CAD build for the part. Positions are in the model's coordinates, mm. Round coordinates to 2 decimals unless told otherwise and drop trailing zeros. Order: outer loops, then holes, each group sorted by start corner. A loop starts at its lowest first (then second) coordinate and runs counter-clockwise, first axis right, second up.
```python
from build123d import *

# Parameters (mm, degrees)
SKETCH2_W           = 73
SKETCH2_H           = 13
SKETCH2_R           = 3.9
SKETCH2_R_2         = 3.95
SKETCH2_R_3         = 4
SKETCH2_R_4         = 4.05
SKETCH2_R_5         = 4.1
SKETCH2_R_6         = 4.15
SKETCH2_R_7         = 4.2
BOSS_EXTRUDE1_DEPTH = 5
FILLET1_R           = 5


with BuildPart() as part:
    # Sketch2 → Boss-Extrude1 (new body)
    with BuildSketch(Plane(origin=(0, 0, 0), x_dir=(1, 0, 0), z_dir=(0, 1, 0))):
        with Locations((30, 0)):
            Rectangle(SKETCH2_W, SKETCH2_H)
        Circle(SKETCH2_R, mode=Mode.SUBTRACT)
        with Locations((10, 0)):
            Circle(SKETCH2_R_2, mode=Mode.SUBTRACT)
        with Locations((20, 0)):
            Circle(SKETCH2_R_3, mode=Mode.SUBTRACT)
        with Locations((30, 0)):
            Circle(SKETCH2_R_4, mode=Mode.SUBTRACT)
        with Locations((40, 0)):
            Circle(SKETCH2_R_5, mode=Mode.SUBTRACT)
        with Locations((50, 0)):
            Circle(SKETCH2_R_6, mode=Mode.SUBTRACT)
        with Locations((60, 0)):
            Circle(SKETCH2_R_7, mode=Mode.SUBTRACT)
    extrude(amount=BOSS_EXTRUDE1_DEPTH)

    # Fillet1
    fillet1_edges = [part.edges().sort_by_distance(p)[0] for p in [
        (-6.5, 2.5, -6.5),
        (-6.5, 2.5, 6.5),
    ]]
    fillet(fillet1_edges, radius=FILLET1_R)


solid = part.part
```
1. Cut at D-D, the plane x = 50. Write the cut outline in (y, z).
2. Cut at C-C, the plane y = 4. Write the cut outline in (x, z).
3. Cut at A-A, the plane x = 40. Write the cut outline in (y, z).
4. Cut at B-B, the plane z = -0.75. Give the number of separate pieces and of enclosed holes in the cut face, and give its area (3 significant figures).
5. Pin check, flat tips, straight feed: P1, Ø5, axis at x = 50, z = 0, coming from the -Y side (3 decimals); P2, Ø6, axis at x = 29.5, z = 3.5, coming from the +Y side. Stop position of each tip, or through.
6. Drill centre lines: line 1 (Z direction, x = 0, y = 3.3); line 2 (Z direction, x = 20, y = 1.55); line 3 (X direction, y = 4.6, z = -4.25). Where is each one in solid material? Low to high.
7. Mould opens along Z. For faces 1 (the face through (-5.07, 2.54, -5)), 2 (the face through (35.904, 2.465, -0.18)), 3 (the face through (29.5, 5, -4.4)) say: released by +Z, released by -Z, zero draft, split by the parting line, or undercut.
Outcome:
1. outline: (0, -6.5) - (5, -6.5) - (5, -4.15) - (0, -4.15) - close; (0, 4.15) - (5, 4.15) - (5, 6.5) - (0, 6.5) - close
2. outline: (-6.5, -1.5) arc R5 ccw to (-1.5, -6.5) - (66.5, -6.5) - (66.5, 6.5) - (-1.5, 6.5) arc R5 ccw to (-6.5, 1.5) - close; hole circle Ø7.8 at (0, 0); hole circle Ø7.9 at (10, 0); hole circle Ø8 at (20, 0); hole circle Ø8.1 at (30, 0); hole circle Ø8.2 at (40, 0); hole circle Ø8.3 at (50, 0); hole circle Ø8.4 at (60, 0)
3. outline: (0, -6.5) - (5, -6.5) - (5, -4.1) - (0, -4.1) - close; (0, 4.1) - (5, 4.1) - (5, 6.5) - (0, 6.5) - close
4. separate pieces: 8
4. enclosed holes: 0
4. area: 86.4 mm2
5. P1: passes through
5. P2: stops at y = 5
6. line 1: z = -6.5 to -3.9, 3.9 to 6.5
6. line 2: z = -6.5 to -4, 4 to 6.5
6. line 3: x = -5.68 to 66.5
7. face 1: released by -Z
7. face 2: undercut
7. face 3: zero draft
